Study the drawing (mm; zero at the part's minimum x, y, z) and answer. Give positions to 0.01 mm unless a question says otherwise; leave off trailing zeros. Write each loop counter-clockwise with the first axis right and the second up, starting at its lowest first coordinate (ties: lowest second). Pieces come first, ordered by that corner, then holes. Notation, with made-up numbers: (84, -29.75) - (103, -29.75) arc R22 cw to (103, -3.75) - close; hole circle Ø4 at (11.25, -13.75). An arc over 180 degrees is marked (long way). Return JSON: item names as keys, results as strings.
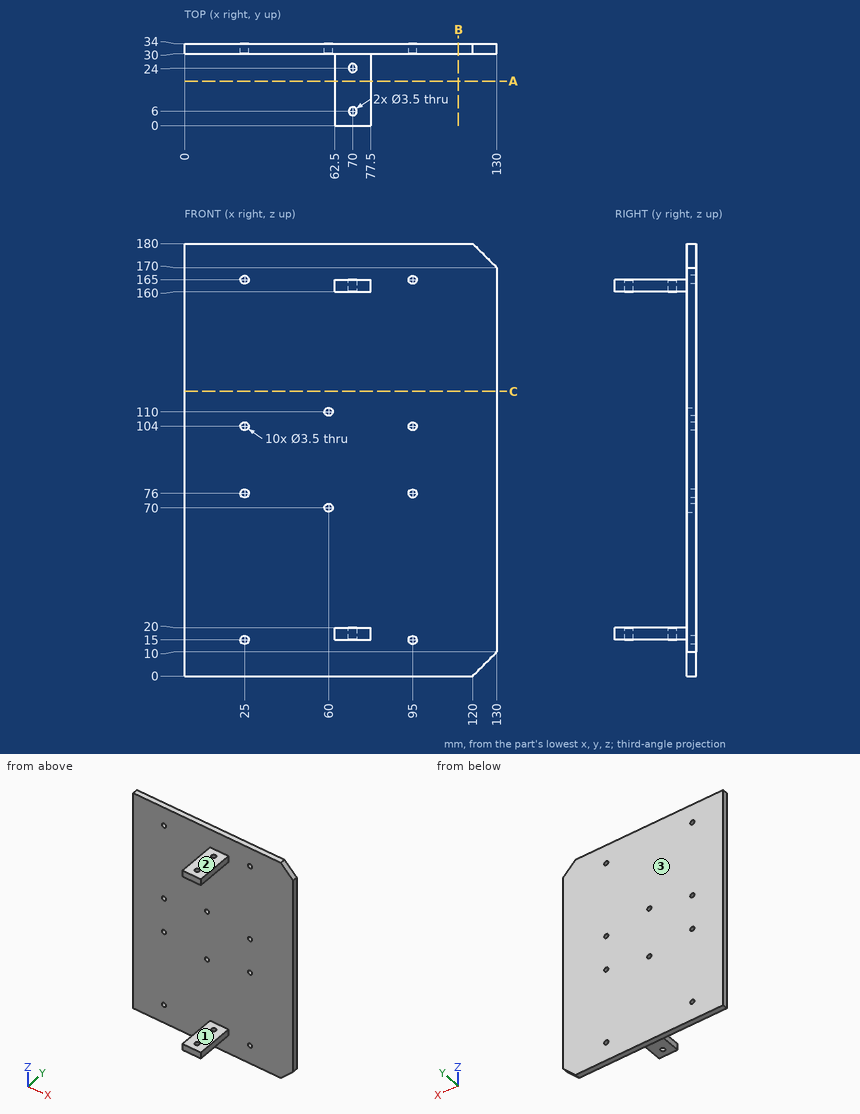
Item 1: A cutting plane is placed at A-A on y = 18.5. Determine the outline of the cut face in (x, z).
Answer below:
{"outline": "(62.5, 15) - (77.5, 15) - (77.5, 20) - (62.5, 20) - close; (62.5, 160) - (77.5, 160) - (77.5, 165) - (62.5, 165) - close"}
Item 2: A cutting plane is placed at C-C on z = 118.5. Determine the outline of the cut face in (x, y).
Answer below:
{"outline": "(0, 30) - (130, 30) - (130, 34) - (0, 34) - close"}
Item 3: A cutting plane is placed at B-B on x = 114. Determine the outline of the cut face in (y, z).
Answer below:
{"outline": "(30, 0) - (34, 0) - (34, 180) - (30, 180) - close"}
Item 4: Consider L1, parallel to X at y = 31.7, z = 15; L2, parallel to Y at x = 70, z = 18; L3, parallel to Y at x = 21, z = 173.5. Determine where each line is inside the solid, lowest interval first.
Answer below:
{"L1": "x = 0 to 23.25, 26.75 to 93.25, 96.75 to 130", "L2": "y = 0 to 4.25, 7.75 to 22.25, 25.75 to 34", "L3": "y = 30 to 34"}
Item 5: Flat-ended cylindrical pins translate along their axes: P1, Ø12, axis at x = 71.5, y = 17, coming from the -Z side; P2, Ø4, axis at x = 70, y = 6, coming from the +Z side; P3, Ø5.5, axis at y = 16, z = 162, coming from the +X side; P4, Ø5.5, axis at x = 95, z = 76, coming from the +Y side. Find the tip coordinate at first contact, or state that the pin passes through.
Answer below:
{"P1": "stops at z = 15", "P2": "stops at z = 165", "P3": "stops at x = 77.5", "P4": "stops at y = 34"}
Item 6: The mould has two halves that part along Z. Classify the marked faces 1, 2 and 3: +Z half, -Z half, draft (parallel to the pull), parting line (faces both ways), or undercut.
Answer below:
{"face 1": "undercut", "face 2": "+Z half", "face 3": "draft"}
